Input: part model. Units: mm. Frame: model coordinates. A direction names the side the tool comes from. Coordinates: 2 decimals unless noted, no trailing zeros. Loops run counter-clockwise (first coordinate to the right, second up) from the corner with the lowest first, then second, coordinate; pieces in that order, holes last. Notation, with made-up numbers: (-15, 72) - (41, 72) arc R19 ccw to (41, 90) - close; hole circle Ø10 at (-13.5, 64). An arc over 180 degrees is marked (long way). Write item = value, one per line. Start each with the question number.
from build123d import *

# Parameters (mm, degrees)
SKETCH2_W           = 154.0002
SKETCH2_H           = 154.0002
BOSS_EXTRUDE1_DEPTH = 4.7625
SKETCH4_R           = 76.2
CUT_EXTRUDE1_DEPTH  = 3.175
SKETCH5_R           = 3.3782
CUT_EXTRUDE2_DEPTH  = 218.841237158
BOSS_EXTRUDE2_DEPTH = 3.175


with BuildPart() as part:
    # Sketch2 → Boss-Extrude1 (new body)
    with BuildSketch(Plane(origin=(0, 0, 0), x_dir=(1, 0, 0), z_dir=(0, 1, 0))):
        with Locations((77.0001, 77.0001)):
            Rectangle(SKETCH2_W, SKETCH2_H)
    extrude(amount=BOSS_EXTRUDE1_DEPTH)

    # Sketch4 → Cut-Extrude1 (cut)
    with BuildSketch(Plane(origin=(0, 4.7625, 0), x_dir=(1, 0, 0), z_dir=(0, 1, 0))):
        with Locations(Location((77.0001, 77.0001, 0), (0, 0, 270))):
            Circle(SKETCH4_R)
    extrude(amount=-CUT_EXTRUDE1_DEPTH, mode=Mode.SUBTRACT)

    # Sketch5 → Cut-Extrude2 (cut, through all)
    with BuildSketch(Plane(origin=(0, 4.7625, 0), x_dir=(1, 0, 0), z_dir=(0, 1, 0))):
        with Locations(Location((6.35, 6.35, 0), (0, 0, 270))):
            Circle(SKETCH5_R)
        with Locations(Location((6.35, 147.6502, 0), (0, 0, 270))):
            Circle(SKETCH5_R)
        with Locations(Location((147.6502, 147.6502, 0), (0, 0, 270))):
            Circle(SKETCH5_R)
        with Locations(Location((147.6502, 6.35, 0), (0, 0, 270))):
            Circle(SKETCH5_R)
    extrude(amount=-CUT_EXTRUDE2_DEPTH, mode=Mode.SUBTRACT)

    # Sketch7 → Boss-Extrude2 (add)
    with BuildSketch(Plane.XZ):
        with BuildLine():
            Line((109.284213593, -89.700088814), (123.348971479, -89.700088814))
            ThreePointArc((123.348971479, -89.700088814), (125.59403551, -88.770152844), (126.523971479, -86.525088814))
            Line((126.523971479, -86.525088814), (126.523971479, -67.475088814))
            ThreePointArc((126.523971479, -67.475088814), (124.341654203, -64.459262889), (120.794707851, -65.589256818))
            Line((120.794707851, -65.589256818), (106.729949965, -84.639256818))
            ThreePointArc((106.729949965, -84.639256818), (106.449769946, -87.955667091), (109.284213593, -89.700088814))
        make_face()
        with BuildLine():
            Line((150.113729365, -64.300088814), (136.048971479, -64.300088814))
            ThreePointArc((136.048971479, -64.300088814), (133.803907449, -65.230024784), (132.873971479, -67.475088814))
            Line((132.873971479, -67.475088814), (132.873971479, -86.525088814))
            ThreePointArc((132.873971479, -86.525088814), (135.056288756, -89.540914739), (138.603235108, -88.410920809))
            Line((138.603235108, -88.410920809), (152.667992994, -69.360920809))
            ThreePointArc((152.667992994, -69.360920809), (152.948173013, -66.044510537), (150.113729365, -64.300088814))
        make_face()
        with BuildLine():
            Line((96.052127079, -88.410920809), (110.116884965, -69.360920809))
            ThreePointArc((110.116884965, -69.360920809), (110.397064984, -66.044510537), (107.562621336, -64.300088814))
            Line((107.562621336, -64.300088814), (93.49786345, -64.300088814))
            ThreePointArc((93.49786345, -64.300088814), (90.748232793, -65.887588814), (90.748232793, -69.062588814))
            ThreePointArc((90.748232793, -69.062588814), (92.875079508, -77.000088814), (90.748232793, -84.937588814))
            ThreePointArc((90.748232793, -84.937588814), (91.758452384, -89.181227768), (96.052127079, -88.410920809))
        make_face()
        with BuildLine():
            Line((25.251556253, -88.788587501), (44.618320403, -69.738587501))
            ThreePointArc((44.618320403, -69.738587501), (45.330145322, -66.272172219), (42.391843659, -64.300088814))
            Line((42.391843659, -64.300088814), (23.025079508, -64.300088814))
            ThreePointArc((23.025079508, -64.300088814), (20.780015478, -65.230024784), (19.850079508, -67.475088814))
            Line((19.850079508, -67.475088814), (19.850079508, -86.525088814))
            ThreePointArc((19.850079508, -86.525088814), (21.797976958, -89.453372327), (25.251556253, -88.788587501))
        make_face()
        with BuildLine():
            Line((58.275818822, -65.211590127), (38.909054672, -84.261590127))
            ThreePointArc((38.909054672, -84.261590127), (38.197229752, -87.728005409), (41.135531416, -89.700088814))
            Line((41.135531416, -89.700088814), (60.502295566, -89.700088814))
            ThreePointArc((60.502295566, -89.700088814), (63.251926223, -88.112588814), (63.251926223, -84.937588814))
            ThreePointArc((63.251926223, -84.937588814), (61.125079508, -77.000088814), (63.251926223, -69.062588814))
            ThreePointArc((63.251926223, -69.062588814), (62.445481153, -64.964181652), (58.275818822, -65.211590127))
        make_face()
    extrude(amount=BOSS_EXTRUDE2_DEPTH)


solid = part.part
Item 1: Ray query, line 1 (Z direction, x = 7, y = 3); line 2 (X direction, y = 4, z = -145); line 3 (Y direction, x = 18, z = -43). Return the intervals inside material, ascending.
Item 2: Cut plane C-C on z = -6.35. Return loops of the section in (x, y).
Item 3: Cut plane B-B on x = 6.35. Return loops of the section in (y, z).
Item 4: Cut plane A-A on y = -1.25. State how many separate pieces and enclosed holes the cut face has, plus the area to 3 significant figures.
Item 5: Access query for faces 1 (the flat face through (113.86, -1.57, -74.98)), 2 (the flat face through (78, 1.588, -78)), 3 (the flat face through (30, -3.175, -74)). Directions: +Z, -Z, +X, -X, +Y, -Y. A direction counts if a zero-diameter tool reaches every point of the face in a straight line with its end or side. Return the directions, or none.
Item 6: Pin query (flat end, axial travel): pin 1 (1.6 mm diameter, centred on x = 146, y = -1.5, fed in from +Z); pin 2 (4 mm diameter, centred on x = 84.5, z = -99, fed in from +Y); pin 3 (3 mm diameter, centred on x = 94, y = 1, fed in from +Z); pin 4 (2.5 mm diameter, centred on y = -2, z = -79, fed in from -X). Return the tip coordinate at first contact, or that it passes through.
Item 7: Cut plane D-D on z = -42. Return loops of the section in (x, y).
Item 8: Pull-direction query (Z, two-part tool) for faces 4 (the flat face through (145.537, -1.565, -79.019)), 5 (the flat face through (42, 4.762, -146)), 6 (the flat face through (103, -2, -79)), 7 (the cylindrical face through (7.365, 2.415, -3.128)); classes: pulls with the +Z half, pulls with the -Z half, needs draft (parallel to the pull), parting line crosses it, or undercut.
Recorded:
q1.line_1 = -154 to -150.97, -144.34 to -107.11, -46.89 to -9.67, -3.03 to 0
q1.line_2 = 0 to 4.26, 8.44 to 42.61, 111.39 to 145.56, 149.75 to 154
q1.line_3 = 0 to 1.59
q2.outline = (0, 0) - (2.97, 0) - (2.97, 4.76) - (0, 4.76) - close; (9.73, 0) - (144.27, 0) - (144.27, 4.76) - (105.55, 4.76) - (105.55, 1.59) - (48.45, 1.59) - (48.45, 4.76) - (9.73, 4.76) - close; (151.03, 0) - (154, 0) - (154, 4.76) - (151.03, 4.76) - close
q3.outline = (0, -154) - (4.76, -154) - (4.76, -151.03) - (0, -151.03) - close; (0, -144.27) - (4.76, -144.27) - (4.76, -105.55) - (1.59, -105.55) - (1.59, -48.45) - (4.76, -48.45) - (4.76, -9.73) - (0, -9.73) - close; (0, -2.97) - (4.76, -2.97) - (4.76, 0) - (0, 0) - close
q4.separate_pieces = 5
q4.enclosed_holes = 0
q4.area = 1,830 mm²
q5.face_1 = -Y
q5.face_2 = +Y
q5.face_3 = +Z, -Z, +X, -X, -Y
q6.pin_1 = -64.3
q6.pin_2 = 1.59
q6.pin_3 = 0
q6.pin_4 = 19.85
q7.outline = (0, 0) - (154, 0) - (154, 4.76) - (144.69, 4.76) - (144.69, 1.59) - (9.31, 1.59) - (9.31, 4.76) - (0, 4.76) - close
q8.face_4 = pulls with the -Z half
q8.face_5 = needs draft
q8.face_6 = undercut
q8.face_7 = undercut
